Source: CAD feature listing. Evaluate the final solid. Frame: model axes, mm. Face numbers are marked on the shaded views. A direction names the side the tool comes from. Give positions to 0.01 mm unless a question says otherwise; leave off trailing zeros. Loops run counter-clockwise (first coordinate to the right, second up) from the corner with the lowest first, then second, coordinate; pieces in that order, holes last. Notation, with made-up numbers: M -21.75,5 L -2.75,5 A13 ccw -2.75,26 Z; hole C 26.5,-6 d1. An arc over 180 degrees is marked long. Put each result on its own line as item: value. Start each with the question number.
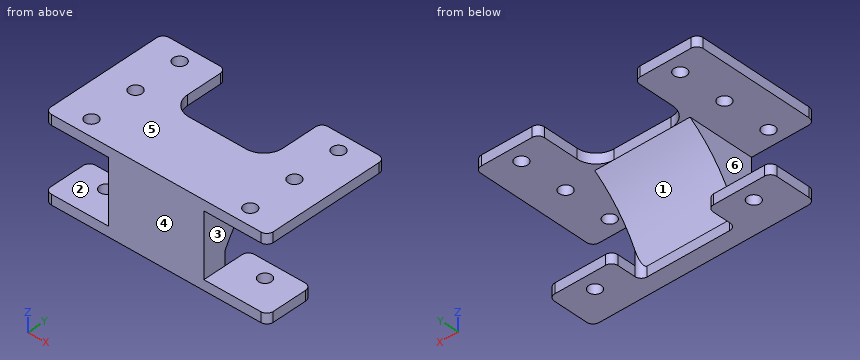
```python
from build123d import *

# Parameters (mm, degrees)
SKETCH1_W             = 25.4
SKETCH1_H             = 50.8
SKETCH1_R             = 2.54
BOSS_EXTRUDE1_DEPTH   = 4
BOSS_EXTRUDE1_2_DEPTH = 4
SKETCH2_W             = 4
SKETCH2_H             = 26.531408834
BOSS_EXTRUDE2_DEPTH   = 38.1
SKETCH3_R             = 2.54
SKETCH3_W             = 19.05
SKETCH3_H             = 6.648533437
BOSS_EXTRUDE3_DEPTH   = 4
FILLET1_R             = 7.62
FILLET2_R             = 2.54


with BuildPart() as part:
    # Sketch1 → Boss-Extrude1 (new body)
    with BuildSketch(Plane.XY):
        with Locations((0, 25.4)):
            Rectangle(SKETCH1_W, SKETCH1_H)
        with Locations((0, 44.45)):
            Circle(SKETCH1_R, mode=Mode.SUBTRACT)
        with Locations((0, 25.4)):
            Circle(SKETCH1_R, mode=Mode.SUBTRACT)
        with Locations((0, 6.35)):
            Circle(SKETCH1_R, mode=Mode.SUBTRACT)
    extrude(amount=BOSS_EXTRUDE1_DEPTH)



with BuildPart() as body_2:
    # Sketch1 → Boss-Extrude1 2 (new body)
    with BuildSketch(Plane.XY):
        with Locations((63.5, 25.4)):
            Rectangle(SKETCH1_W, SKETCH1_H)
        with Locations((63.5, 25.4)):
            Circle(SKETCH1_R, mode=Mode.SUBTRACT)
        with Locations((63.5, 44.45)):
            Circle(SKETCH1_R, mode=Mode.SUBTRACT)
        with Locations((63.5, 6.35)):
            Circle(SKETCH1_R, mode=Mode.SUBTRACT)
    extrude(amount=BOSS_EXTRUDE1_2_DEPTH)


with BuildPart() as part_1:
    add(part.part)

    add(body_2.part)  # Boss-Extrude2 merges body 2
    # Sketch2 → Boss-Extrude2 (add)
    with BuildSketch(Plane.ZY.offset(-50.8)):
        with BuildLine():
            Line((0, 0), (0, 26.531408834))
            ThreePointArc((0, 26.531408834), (-11.179973196, 14.648165434), (-25.4, 6.648533437))
            Line((-25.4, 6.648533437), (-25.4, 0))
            Line((-25.4, 0), (0, 0))
        make_face()
        with Locations((2, 13.265704417)):
            Rectangle(SKETCH2_W, SKETCH2_H)
    extrude(amount=BOSS_EXTRUDE2_DEPTH)

    # Sketch3 → Boss-Extrude3 (add)
    # profile 1 of 3: a face of its own
    with BuildSketch(Plane(origin=(0, 0, -25.4), x_dir=(-1, 0, 0), z_dir=(0, 0, -1))):
        Polygon((-12.7, 6.648533437), (-12.7, 0), (12.7, 0), (12.7, 19.05), (-12.7, 19.05), align=None)
        with Locations(Location((0, 12.7, 0), (0, 0, 90))):
            Circle(SKETCH3_R, mode=Mode.SUBTRACT)
    # profile 2 of 3: a face of its own
    with BuildSketch(Plane(origin=(0, 0, -25.4), x_dir=(-1, 0, 0), z_dir=(0, 0, -1))):
        with Locations((-22.225, 3.324266719)):
            Rectangle(SKETCH3_W, SKETCH3_H)
    # profile 3 of 3: a face of its own
    with BuildSketch(Plane(origin=(0, 0, -25.4), x_dir=(-1, 0, 0), z_dir=(0, 0, -1))):
        Polygon((-76.2, 0), (-31.75, 0), (-31.75, 6.648533437), (-50.8, 6.648533437), (-50.8, 19.05), (-76.2, 19.05), align=None)
        with Locations(Location((-63.5, 12.7, 0), (0, 0, 90))):
            Circle(SKETCH3_R, mode=Mode.SUBTRACT)
    extrude(amount=BOSS_EXTRUDE3_DEPTH)

    # Fillet1
    # the kernel refuses this fillet: 7.62 mm, written as the material it adds along each edge
    with BuildSketch(Plane(origin=(12.7, 26.531408834, 4), x_dir=(0, 1, 0), z_dir=(0, 0, -1)), Plane(origin=(50.8, 26.531408834, 4), x_dir=(-1, 0, 0), z_dir=(0, 0, -1))) as fillet1_piece_1:
        with BuildLine():
            CenterArc((FILLET1_R, FILLET1_R), FILLET1_R, 180, 90)
            Line((0, FILLET1_R), (0, 0))
            Line((0, 0), (FILLET1_R, 0))
        make_face()
    extrude(amount=4)

    # Fillet2
    # the kernel refuses this fillet: 2.54 mm, written as the material it adds along each edge
    with BuildSketch(Plane(origin=(12.7, 6.648533437, -19.05), x_dir=(1, 0, 0), z_dir=(0, 0, -1))) as fillet2_piece_1:
        with BuildLine():
            CenterArc((FILLET2_R, -FILLET2_R), FILLET2_R, 90, 90)
            Line((0, -FILLET2_R), (0, 0))
            Line((0, 0), (FILLET2_R, 0))
        make_face()
    extrude(amount=10.35)
    with BuildSketch(Plane(origin=(50.8, 6.648533437, -19.05), x_dir=(-1, 0, 0), z_dir=(0, 0, -1))) as fillet2_piece_2:
        with BuildLine():
            CenterArc((FILLET2_R, FILLET2_R), FILLET2_R, 180, 90)
            Line((0, FILLET2_R), (0, 0))
            Line((0, 0), (FILLET2_R, 0))
        make_face()
    extrude(amount=10.35)
    # the kernel refuses this fillet: 2.54 mm, written as the material it takes off along each edge
    with BuildSketch(Plane(origin=(12.7, 50.8, -6.35), x_dir=(-1, 0, 0), z_dir=(0, 0, 1)), Plane(origin=(-12.7, 0, -6.35), x_dir=(1, 0, 0), z_dir=(0, 0, 1)), Plane(origin=(76.2, 0, -6.35), x_dir=(0, 1, 0), z_dir=(0, 0, 1)), Plane(origin=(76.2, 50.8, -6.35), x_dir=(-1, 0, 0), z_dir=(0, 0, 1)), Plane(origin=(-12.7, 19.05, -19.05), x_dir=(1, 0, 0), z_dir=(0, 0, -1)), Plane(origin=(12.7, 19.05, -19.05), x_dir=(0, -1, 0), z_dir=(0, 0, -1)), Plane(origin=(50.8, 19.05, -19.05), x_dir=(1, 0, 0), z_dir=(0, 0, -1)), Plane(origin=(76.2, 0, -19.05), x_dir=(-1, 0, 0), z_dir=(0, 0, -1))) as fillet2_2_piece_1:
        with BuildLine():
            CenterArc((FILLET2_R, FILLET2_R), FILLET2_R, 180, 90)
            Line((0, FILLET2_R), (0, 0))
            Line((0, 0), (FILLET2_R, 0))
        make_face()
    extrude(amount=16.7, mode=Mode.SUBTRACT)
    with BuildSketch(Plane(origin=(-12.7, 50.8, -6.35), x_dir=(1, 0, 0), z_dir=(0, 0, 1)), Plane(origin=(50.8, 50.8, -6.35), x_dir=(1, 0, 0), z_dir=(0, 0, 1)), Plane(origin=(-12.7, 0, -19.05), x_dir=(1, 0, 0), z_dir=(0, 0, -1)), Plane(origin=(76.2, 19.05, -19.05), x_dir=(-1, 0, 0), z_dir=(0, 0, -1))) as fillet2_2_piece_2:
        with BuildLine():
            CenterArc((FILLET2_R, -FILLET2_R), FILLET2_R, 90, 90)
            Line((0, -FILLET2_R), (0, 0))
            Line((0, 0), (FILLET2_R, 0))
        make_face()
    extrude(amount=16.7, mode=Mode.SUBTRACT)


solid = part_1.part
```
1. Section C-C, the plane y = 25.4. Output: boundary loops of the cut face in (x, z), plus the area to 3 significant figures.
2. Ray query, line 1 (X direction, y = 12.7, z = -26.95); line 2 (Y direction, x = 0, z = 1); line 3 (Z direction, x = 10.5, y = 10.5). Return the intervals inside material, ascending.
3. Section B-B, the plane x = 63.5. Output: boundary loops of the cut face in (y, z), plus the area to 3 significant figures.
4. Section A-A, the plane y = 44.45. Output: boundary loops of the cut face in (x, z), plus the area to 3 significant figures.
5. Pull-direction query (Z, two-part tool) for the marked faces 4, 5 and 6; classes: released by +Z, released by -Z, zero draft, split by the parting line, or undercut.
6. Set-up query: the marked faces 1, 2 and 3. Return all of +Z, -Z, +X, -X, +Y, -Y with unobstructed straight access to the full face (end or side cutting, diameter ignored); none if empty.
7. Section D-D, the plane y = 12.7. Output: boundary loops of the cut face in (x, z).
8. Contact query for flat-ended pins moving along their axis: pin 1 (1.5 mm diameter, centred on x = 34.5, y = 25, fed in from -Z); pin 2 (10 mm diameter, centred on x = 9, y = 29, fed in from -Z); pin 3 (4.5 mm diameter, centred on x = 0, y = 6.35, fed in from +Z); pin 4 (8 mm diameter, centred on x = 0, y = 25.4, fed in from +Z). Output: stop coordinate, or through.
Results found:
1. outline: M -12.7,0 L -2.54,0 L -2.54,4 L -12.7,4 Z; M 2.54,0 L 12.7,0 L 12.7,-0.8 L 50.8,-0.8 L 50.8,0 L 60.96,0 L 60.96,4 L 2.54,4 Z; M 66.04,0 L 76.2,0 L 76.2,4 L 66.04,4 Z
1. area: 345 mm²
2. line 1: -12.7 to -2.54, 2.54 to 12.7, 50.8 to 60.96, 66.04 to 76.2
2. line 2: 0 to 3.81, 8.89 to 22.86, 27.94 to 41.91, 46.99 to 50.8
2. line 3: -29.4 to -25.4, 0 to 4
3. outline: M 0,-29.4 L 10.16,-29.4 L 10.16,-25.4 L 0,-25.4 Z; M 0,0 L 3.81,0 L 3.81,4 L 0,4 Z; M 8.89,0 L 22.86,0 L 22.86,4 L 8.89,4 Z; M 15.24,-29.4 L 19.05,-29.4 L 19.05,-25.4 L 15.24,-25.4 Z; M 27.94,0 L 41.91,0 L 41.91,4 L 27.94,4 Z; M 46.99,0 L 50.8,0 L 50.8,4 L 46.99,4 Z
3. area: 198 mm²
4. outline: M -12.7,0 L -2.54,0 L -2.54,4 L -12.7,4 Z; M 2.54,0 L 12.7,0 L 12.7,4 L 2.54,4 Z; M 50.8,0 L 60.96,0 L 60.96,4 L 50.8,4 Z; M 66.04,0 L 76.2,0 L 76.2,4 L 66.04,4 Z
4. area: 163 mm²
5. face 4: zero draft
5. face 5: released by +Z
5. face 6: undercut
6. face 1: -Z, +Y
6. face 2: -X, +Y, -Y
6. face 3: +X, +Y, -Y
7. outline: M -12.7,-29.4 L -2.54,-29.4 L -2.54,-25.4 L -12.7,-25.4 Z; M -12.7,0 L 12.7,0 L 12.7,-13.83 L 50.8,-13.83 L 50.8,0 L 76.2,0 L 76.2,4 L -12.7,4 Z; M 2.54,-29.4 L 12.7,-29.4 L 12.7,-25.4 L 2.54,-25.4 Z; M 50.8,-29.4 L 60.96,-29.4 L 60.96,-25.4 L 50.8,-25.4 Z; M 66.04,-29.4 L 76.2,-29.4 L 76.2,-25.4 L 66.04,-25.4 Z
8. pin 1: z = -1.66
8. pin 2: z = -0.63
8. pin 3: z = -25.4
8. pin 4: z = 4
